Verification items for this drawing (mm, ordinates from the low corner). A direction names the side the tool comes from. Round coordinates to 2 decimals unless told otherwise and drop trailing zeros. Loops run counter-clockwise (first coordinate to the right, second up) from the corner with the lowest first, then second, coordinate; pieces in that order, holes last. Notation, with made-up numbers: (81.5, -20.75) - (124.5, -20.75) arc R33 ccw to (124.5, 7.25) - close; hole circle Ø8 at (-36, -12.75). An arc over 180 degrees is marked (long way). Answer in a Markdown table with one row per item. Add a question column.
(1) Cross-section at B-B on x = 21. Enter the section's corners in (y, z).
(2) Cross-section at C-C on z = 25.5. Enter the section's corners in (x, y).
(3) Mould release check, pull along X, two halves, no side actions. Record for the marked faces 1, 2 and 3: +X half, -X half, draft (parallel to the pull), parting line (faces both ways), or undercut.
(4) Cross-section at D-D on y = 3.5. Enter the section's corners in (x, z), then the cut area to 3 significant figures.
(5) Thickness scan on line 1 along Y through (x, z) = (21, 27.75); line 2 along Z through (x, y) = (14, 44); line 3 along X through (y, z) = (31.5, 22.5). Record the ranges inside material, lowest first.
(6) Cross-section at A-A on y = 30. Enter the section's corners in (x, z).
(7) Access from +Z, -Z, +X, -X, +Y, -Y to the whole of each face (thin tool, end or side, straight path). Record for the marked faces 4, 5 and 6.
(8) Gauge pin test, flat end, axial feed: pin 1 (13 mm diameter, centred on x = 21, y = 9.5, fed in from -Z). Record the tip position at first contact, or that the pin passes through.
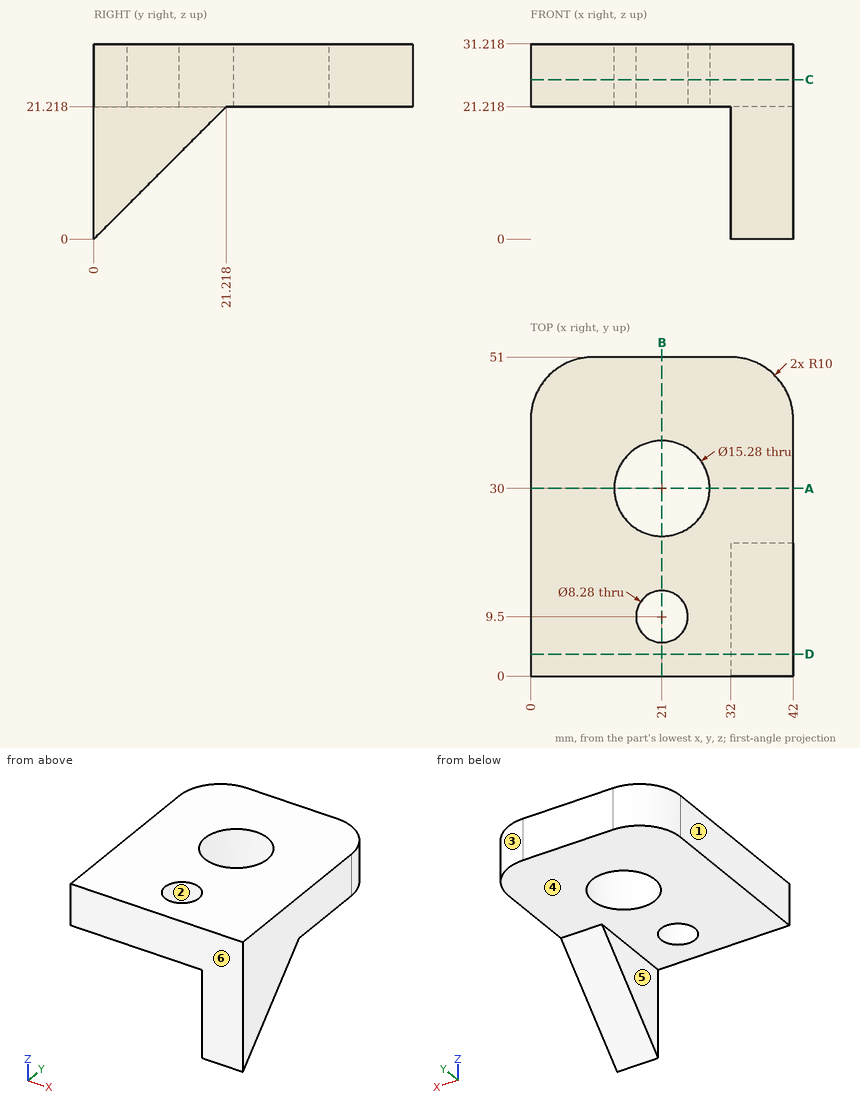
Answers:
| question | item | result |
|---|---|---|
| 1 | outline | (0, 21.22) - (5.36, 21.22) - (5.36, 31.22) - (0, 31.22) - close; (13.64, 21.22) - (22.36, 21.22) - (22.36, 31.22) - (13.64, 31.22) - close; (37.64, 21.22) - (51, 21.22) - (51, 31.22) - (37.64, 31.22) - close |
| 2 | outline | (0, 0) - (42, 0) - (42, 41) arc R10 ccw to (32, 51) - (10, 51) arc R10 ccw to (0, 41) - close; hole circle Ø15.28 at (21, 30); hole circle Ø8.28 at (21, 9.5) |
| 3 | face 1 | -X half |
| 3 | face 2 | undercut |
| 3 | face 3 | +X half |
| 4 | outline | (0, 21.22) - (32, 21.22) - (32, 3.5) - (42, 3.5) - (42, 31.22) - (0, 31.22) - close |
| 4 | area | 597 mm^2 |
| 5 | line 1 | y = 0 to 5.36, 13.64 to 22.36, 37.64 to 51 |
| 5 | line 2 | z = 21.22 to 31.22 |
| 5 | line 3 | x = 0 to 13.51, 28.49 to 42 |
| 6 | outline | (0, 21.22) - (13.36, 21.22) - (13.36, 31.22) - (0, 31.22) - close; (28.64, 21.22) - (42, 21.22) - (42, 31.22) - (28.64, 31.22) - close |
| 7 | face 4 | -Z, -X, +Y |
| 7 | face 5 | -Z, -X, +Y, -Y |
| 7 | face 6 | +Z, -Z, +X, -X, -Y |
| 8 | pin 1 | stops at z = 21.22 |
